Can you work these out from the model? Positions are in its coordinate system, mm. Give positions to 0.01 mm unless a question says otherwise; leave off trailing zeros. Order: outer loops, then holes, each group sorted by start corner. A loop starts at its lowest first (then second) coordinate and runs counter-clockwise, first axis right, second up. Notation, with made-up numbers: (15, 15) - (29, 15) arc R31 cw to (29, 50) - close; hole circle Ø10 at (73.5, -21). An arc over 180 degrees is marked (long way). Answer as CSV lines item,"result".
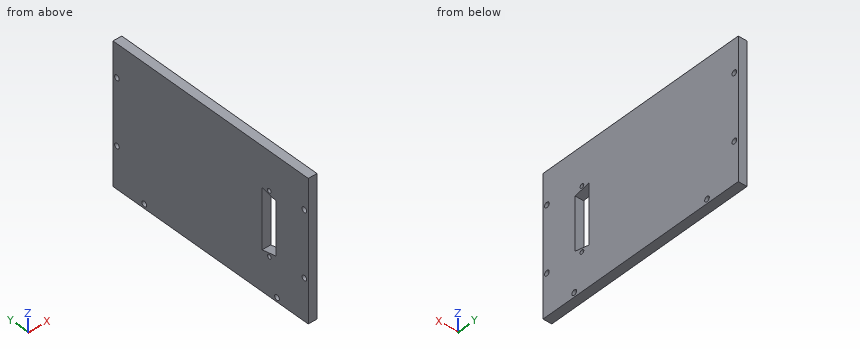
```python
from build123d import *

# Parameters (mm, degrees)
SKETCH1_W             = 101.6
SKETCH1_H             = 158.75
BOSS_EXTRUDE1_DEPTH   = 6.35
SKETCH2_R             = 1.5
CUT_EXTRUDE1_DEPTH    = 95.452914857
CUT_EXTRUDE2_DEPTH    = 95.452914857
F_6_CLEARANCE_HOLE1_D = 3.7973


with BuildPart() as part:
    # Sketch1 → Boss-Extrude1 (new body)
    with BuildSketch(Plane(origin=(0, 0, 0), x_dir=(0, 0, -1), z_dir=(1, 0, 0))):
        Rectangle(SKETCH1_W, SKETCH1_H)
    extrude(amount=BOSS_EXTRUDE1_DEPTH)

    # Sketch2 → Cut-Extrude1 (cut, through all)
    with BuildSketch(Plane(origin=(6.35, 0, 0), x_dir=(0, 0, -1), z_dir=(1, 0, 0))):
        with Locations((23, -47.725)):
            Circle(SKETCH2_R)
        with Locations((-23, -47.725)):
            Circle(SKETCH2_R)
    extrude(amount=-CUT_EXTRUDE1_DEPTH, mode=Mode.SUBTRACT)

    # Sketch3 → Cut-Extrude2 (cut, through all)
    with BuildSketch(Plane(origin=(6.35, 0, 0), x_dir=(0, 0, -1), z_dir=(1, 0, 0))):
        Polygon((-21.709996503, -41.820570024), (-19.255793917, -53.208070024), (19.255793917, -53.208070024), (21.709996503, -41.820570024), align=None)
    extrude(amount=-CUT_EXTRUDE2_DEPTH, mode=Mode.SUBTRACT)

    # #6 Clearance Hole1 (through all)
    with Locations(Plane(origin=(6.35, 0, 0), x_dir=(0, 0, -1), z_dir=(1, 0, 0))):
        with Locations((47.625, -53.975), (-26.9875, 76.2), (20.6375, 76.2), (-26.9875, -76.2), (20.6375, -76.2), (47.625, 53.975)):
            Hole(F_6_CLEARANCE_HOLE1_D / 2)


solid = part.part
```
1) I need wall thicknesses on line 1 along Y through (x, z) = (3.75, -6) (3 decimals); line 2 along Z through (x, y) = (1.75, -76.2); line 3 along Y through (x, z) = (4, -23) (3 decimals). Which ranges of each line are inside material? Lowest first, please. Write a range as [from, to].
Answer block:
line 1,"[-79.375, -53.208], [-41.821, 79.375]"
line 2,"[-50.8, -22.54], [-18.74, 25.09], [28.89, 50.8]"
line 3,"[-79.375, -49.225], [-46.225, 79.375]"
2) I want a section at B-B on y = -76.2. Write out the boundary of the cut face in (x, z).
Answer block:
outline,"(0, -50.8) - (6.35, -50.8) - (6.35, -22.54) - (0, -22.54) - close; (0, -18.74) - (6.35, -18.74) - (6.35, 25.09) - (0, 25.09) - close; (0, 28.89) - (6.35, 28.89) - (6.35, 50.8) - (0, 50.8) - close"
3) I want a section at C-C on x = 3.25. Count the separate pieces of the cut face and the enclosed holes in it, plus the area to 3 significant figures.
Answer block:
separate pieces,"1"
enclosed holes,"9"
area,"15,600 mm2"
4) I want a section at A-A on z = -16.5. Write out the boundary of the cut face in (x, y) (3 decimals).
Answer block:
outline,"(0, -79.375) - (6.35, -79.375) - (6.35, -53.208) - (0, -53.208) - close; (0, -41.821) - (6.35, -41.821) - (6.35, 79.375) - (0, 79.375) - close"
5) I'm going to push a flat-ended pin straight in: P1, Ø6, axis at y = 53.975, z = -47.625, coming from the +X side. Where does the tip first touch, or does it pass through?
Answer block:
P1,"x = 6.35"
